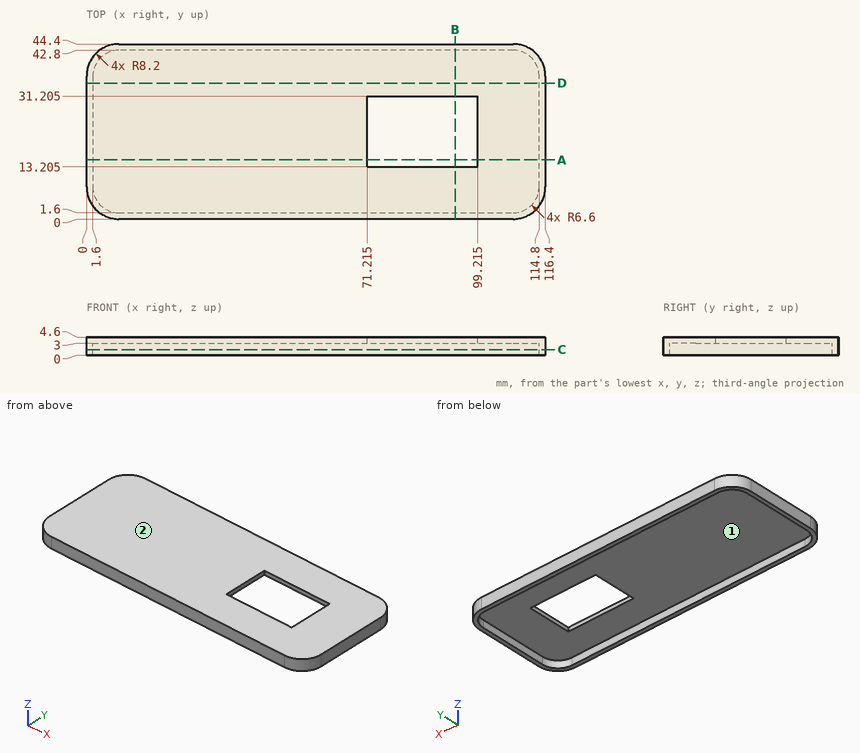
Verification items for this drawing (mm, ordinates from the low corner). Give positions to 0.01 mm unless a question says otherwise; leave off trailing zeros. Loops run counter-clockwise (first coordinate to the right, second up) from the corner with the lowest first, then second, coordinate; pieces in that order, holes last. Notation, with made-up numbers: M 77.5,36 L 113.5,36 A7 ccw 113.5,49 Z; hole C -18.75,83 d11. An arc over 180 degrees is marked long. Answer as a JSON object with one key per item and string values. Group by question number.
Q1. Go/stop test with flat-tipped pins: P1, Ø10, axis at x = 19, y = 15, coming from the -Z side; P2, Ø2, axis at y = 38.5, z = 1, coming from the +X side. Record where each tip stops, or that it passes through.
Q2. Cross-section at D-D on y = 34.5. Record the cut outline in (x, z), then the cut area to 3 significant figures.
Q3. Release check for a two-part mould opening along X. For the marked faces 1 and 2 record: released by +X, released by -X, zero draft, split by the parting line, or undercut.
Q4. Cross-section at B-B on x = 93.5. Record the cut outline in (y, z) (1 decimal).
Q5. Material ranges on line 1 along X through (y, z) = (15, 3.3) (1 decimal); line 2 along Y through (x, z) = (24, 2.55); line 3 along X through (y, z) = (21.5, 1.2), recorded low to high. Write a range as [from, to].
Q6. Cross-section at C-C on z = 1.4. Record the cut outline in (x, y), then the cut area to 3 significant figures.
Q7. Cross-section at A-A on y = 15. Record the cut outline in (x, z) (1 decimal), then the cut area to 3 significant figures.
Evaluation:
{
 "1": {"P1": "stops at z = 3", "P2": "stops at x = 116.3"},
 "2": {"outline": "M 0,0 L 1.6,0 L 1.6,3 L 114.8,3 L 114.8,0 L 116.4,0 L 116.4,4.6 L 0,4.6 Z", "area": "196 mm2"},
 "3": {"face 1": "undercut", "face 2": "zero draft"},
 "4": {"outline": "M 0,0 L 1.6,0 L 1.6,3 L 13.2,3 L 13.2,4.6 L 0,4.6 Z; M 31.2,3 L 42.8,3 L 42.8,0 L 44.4,0 L 44.4,4.6 L 31.2,4.6 Z"},
 "5": {"line 1": "x = [0, 71.2], [99.2, 116.4]", "line 2": "y = [0, 1.6], [42.8, 44.4]", "line 3": "x = [0, 1.6], [114.8, 116.4]"},
 "6": {"outline": "M 0,8.2 A8.2 ccw 8.2,0 L 108.2,0 A8.2 ccw 116.4,8.2 L 116.4,36.2 A8.2 ccw 108.2,44.4 L 8.2,44.4 A8.2 ccw 0,36.2 Z; hole M 1.6,8.2 A6.6 ccw 8.2,1.6 L 108.2,1.6 A6.6 ccw 114.8,8.2 L 114.8,36.2 A6.6 ccw 108.2,42.8 L 8.2,42.8 A6.6 ccw 1.6,36.2 Z", "area": "484 mm2"},
 "7": {"outline": "M 0,0 L 1.6,0 L 1.6,3 L 71.2,3 L 71.2,4.6 L 0,4.6 Z; M 99.2,3 L 114.8,3 L 114.8,0 L 116.4,0 L 116.4,4.6 L 99.2,4.6 Z", "area": "151 mm2"}
}
